from build123d import *

# Parameters (mm, degrees)
BOSS_EXTRUDE1_DEPTH      = 30.48
BOSS_EXTRUDE1_DEPTH_BACK = 23.495
SKETCH1_R                = 6.35
SKETCH2_R                = 8.89
BOSS_EXTRUDE2_DEPTH      = 1.27
SKETCH4_R                = 7.14375
BOSS_EXTRUDE3_DEPTH      = 15.495
SKETCH5_R                = 3.571875
CUT_EXTRUDE1_DEPTH       = 56.41989557


with BuildPart() as part:
    # Sketch1 → Boss-Extrude1 (new, two sides: drawn at the far end of the back side and taken through both)
    with BuildSketch(Plane.XY.offset(-BOSS_EXTRUDE1_DEPTH_BACK)):
        Circle(SKETCH1_R)
    extrude(amount=BOSS_EXTRUDE1_DEPTH + BOSS_EXTRUDE1_DEPTH_BACK)

    # Sketch2 → Boss-Extrude2 (add, symmetric)
    with BuildSketch(Plane.XY):
        Circle(SKETCH2_R)
    extrude(amount=BOSS_EXTRUDE2_DEPTH, both=True)

    # Sketch4 → Boss-Extrude3 (add)
    with BuildSketch(Plane.XY):
        Circle(SKETCH4_R)
    extrude(amount=-BOSS_EXTRUDE3_DEPTH)

    # Sketch5 → Cut-Extrude1 (cut, through all)
    with BuildSketch(Plane.XY.offset(30.48)):
        Circle(SKETCH5_R)
    extrude(amount=-CUT_EXTRUDE1_DEPTH, mode=Mode.SUBTRACT)


solid = part.part
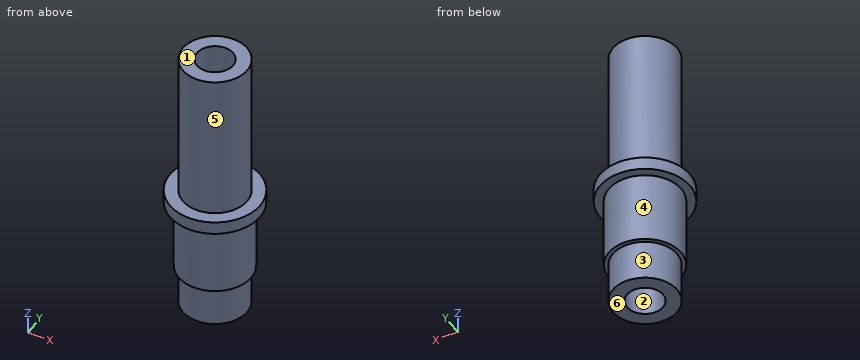
Geometry check sheet. Reference: the model listing, model coordinates, mm. Face numbers are marked on the shaded views. A direction names the side the tool comes from. Coordinates: 2 decimals unless noted, no trailing zeros. Order: outer loops, then holes, each group sorted by start corner. A loop starts at its lowest first (then second) coordinate and runs counter-clockwise, first axis right, second up. Notation, with made-up numbers: (-14, 56) - (29, 56) arc R24 ccw to (29, 95) - close; hole circle Ø5 at (-24.5, 56). An arc over 180 degrees is marked (long way). One line per item, written item: value.
(1) Depth check by flat-ended pin: pin 1 Ø4 at (y, z) = (-6, 23) entering from -X; pin 2 Ø3 at (x, z) = (-1.5, 19) entering from +Y. Enter the tip coordinate at first touch or a pass-through.
Data:
pin 1: stops at x = -4.93
pin 2: stops at y = 6.35
(2) Release check for a two-part mould opening along X. For the marked faces 1, 2 and 3 record: +X half, -X half, draft (parallel to the pull), parting line (faces both ways), or undercut.
Data:
face 1: draft
face 2: undercut
face 3: parting line
(3) Sectioned sample at C-C (z = 7). Enter the section's corners in (x, y).
Data:
outline: circle Ø12.7 at (0, 0); hole circle Ø7.14 at (0, 0)
(4) Sectioned sample at D-D (y = -4.75). Enter the section's corners in (x, z) (3 decimals).
Data:
outline: (-7.515, -1.27) - (-5.336, -1.27) - (-5.336, -15.495) - (-4.214, -15.495) - (-4.214, -23.495) - (4.214, -23.495) - (4.214, -15.495) - (5.336, -15.495) - (5.336, -1.27) - (7.515, -1.27) - (7.515, 1.27) - (4.214, 1.27) - (4.214, 30.48) - (-4.214, 30.48) - (-4.214, 1.27) - (-7.515, 1.27) - close
(5) Sectioned sample at A-A (y = 0). Enter the section's corners in (x, z) (3 decimals), and give its area (3 significant figures).
Data:
outline: (-8.89, -1.27) - (-7.144, -1.27) - (-7.144, -15.495) - (-6.35, -15.495) - (-6.35, -23.495) - (-3.572, -23.495) - (-3.572, 30.48) - (-6.35, 30.48) - (-6.35, 1.27) - (-8.89, 1.27) - close; (3.572, -23.495) - (6.35, -23.495) - (6.35, -15.495) - (7.144, -15.495) - (7.144, -1.27) - (8.89, -1.27) - (8.89, 1.27) - (6.35, 1.27) - (6.35, 30.48) - (3.572, 30.48) - close
area: 335 mm^2
(6) Access from +Z, -Z, +X, -X, +Y, -Y to the whole of each face (thin tool, end or side, straight path). Record for the marked faces 4, 5 and 6.
Data:
face 4: -Z
face 5: +Z
face 6: -Z, +X, -X, +Y, -Y
(7) Thickness scan on probe 1 along Y at (x, z) = (0, 13); probe 2 along Z at (x, y) = (-8, 1); probe 3 along Y at (x, z) = (0, -0.5). Record the ranges inside material, lowest first. Write a range as from..to.
Data:
probe 1: y = -6.35..-3.57, 3.57..6.35
probe 2: z = -1.27..1.27
probe 3: y = -8.89..-3.57, 3.57..8.89
